Read the model definition and answer for the solid it produces. Units are mm, in the model's axes. Round coordinates to 2 decimals unless told otherwise and drop trailing zeros. Loops run counter-clockwise (first coordinate to the right, second up) from the corner with the lowest first, then second, coordinate; pieces in that order, holes last. Notation, with made-up numbers: M 41.25,-21 L 95.25,-21 A19 ccw 95.25,2 Z; hole C -21.75,-24.5 d1. An arc over 180 degrees is marked long. Write each question's results on one line, items separated by ' | '.
from build123d import *

# Parameters (mm, degrees)
F1_DEPTH = 25.4
F2_R     = 12.0698506183
F3_DEPTH = 100.2924419072


with BuildPart() as f1:
    # F0 (on Right) → F1 (new body)
    with BuildSketch(Plane.YZ):
        with BuildLine():
            Line((15.5100870162, 42.3829037865), (15.5131848078, 0))
            Line((15.5131848078, 0), (58.4104247391, 0))
            add(Edge.make_bspline(
                [(-13.0677023463, 80.5449451426), (5.0006115747, 84.8992469104), (47.0210201722, 95.025788891), (54.2753672082, 34.5002323585), (58.4104247391, 0)],
                knots=[0, 0, 0, 0, 0.4299890107, 1, 1, 1, 1], degree=3))
            ThreePointArc((-13.0677023463, 80.5449451426), (7.1384855982, 72.1769982749), (15.509386141, 51.9720337826))
            Line((15.509386141, 51.9720337826), (15.5100870162, 42.3829037865))
        make_face()
        with BuildLine():
            Line((58.4104247391, 0), (15.5131848078, 0))
            Line((15.5131848078, 0), (15.5100870162, 42.3829037865))
            Line((15.5100870162, 42.3829037865), (15.509386141, 51.9720337826))
            ThreePointArc((15.509386141, 51.9720337826), (7.1384855982, 72.1769982749), (-13.0677023463, 80.5449451426))
            Line((-13.0677023463, 80.5449451426), (-52.7544449859, 80.542044415))
            Line((-52.7544449859, 80.542044415), (-52.9602865575, 64.6042414004))
            Line((-52.9602865575, 64.6042414004), (-28.5797221689, 64.6060233903))
            ThreePointArc((-28.5797221689, 64.6060233903), (-8.3735342243, 56.2380765226), (-0.0026336815, 36.0331120303))
            Line((-0.0026336815, 36.0331120303), (0, 0))
            Line((0, 0), (0, -19.7412725538))
            Line((0, -19.7412725538), (58.4104247391, -19.7412725538))
            Line((58.4104247391, -19.7412725538), (58.4104247391, 0))
        make_face()
    extrude(amount=F1_DEPTH)

    # F2 (on face) → F3 (cut, through all)
    with BuildSketch(Plane(origin=(0, -0.0058871476, 80.5458998384), x_dir=(1, 0, 0), z_dir=(0, -7.30906e-05, 0.9999999973))):
        with Locations((12.6999961212, -33.7315686047)):
            Circle(F2_R)
    extrude(amount=-F3_DEPTH, mode=Mode.SUBTRACT)


solid = f1.part
Item 1: Flat-ended cylindrical pins translate along their axes: pin 1 (10 mm diameter, centred on x = 12.5, z = -6, fed in from -Y); pin 2 (12 mm diameter, centred on x = 18.5, y = -41.5, fed in from -Z); pin 3 (5 mm diameter, centred on x = 10, y = 28.5, fed in from +Z). Find the tip coordinate at first contact, or state that the pin passes through.
Outcome:
pin 1: stops at y = 0 | pin 2: stops at z = 64.6 | pin 3: stops at z = 84.58
Item 2: The mould has two halves that part along X. Classify faces 1 (the face through (13, 29, -19.741)), 2 (the face through (23.85, -38.36, 72.27)), 3 (the face through (25.4, 14, 38)), 4 (the face through (0, 14, 38)): pulls with the +X half, pulls with the -X half, needs draft (parallel to the pull), parting line crosses it, or undercut.
Outcome:
face 1: needs draft | face 2: undercut | face 3: pulls with the +X half | face 4: pulls with the -X half
Item 3: The part is cut by section A-A (z = -9). Determine the outline of the cut face in (x, y), plus the area to 3 significant figures.
Outcome:
outline: M 0,0 L 25.4,0 L 25.4,58.41 L 0,58.41 Z | area: 1,480 mm2
Item 4: The part is cut by section B-B (y = -14.5). Determine the outline of the cut face in (x, z), plus the area to 3 significant figures.
Outcome:
outline: M 0,60.9 L 25.4,60.9 L 25.4,80.54 L 0,80.54 Z | area: 499 mm2
Item 5: Straight lines are drawn through the part: line 1 (Y direction, x = 19.5, z = 74); line 2 (Z direction, x = 12.75, y = 17); line 3 (Y direction, x = 17, z = 32). For each, find the intervals that lie inside material, in ascending order.
Outcome:
line 1: y = -52.84 to -43.71, -23.76 to 40.84 | line 2: z = -19.74 to 85.57 | line 3: y = 0 to 54.13
